Can you work these out from the model? Positions are in its coordinate system, mm. A direction names the side the tool comes from. Coordinates: 2 decimals unless noted, no trailing zeros. Loops run counter-clockwise (first coordinate to the right, second up) from the corner with the lowest first, then second, coordinate; pieces in that order, holes last.
```python
from build123d import *

# Parameters (mm, degrees)
SKETCH1_R                             = 31.75
BOSS_EXTRUDE1_DEPTH                   = 15.24
FILLET1_R                             = 5.08
CUT_EXTRUDE2_DEPTH                    = 74.66
F_1_4_0_26_DIAMETER_HOLE1_D           = 6.604
F_1_4_0_26_DIAMETER_HOLE1_DEPTH       = 25.4
F_1_4_0_26_DIAMETER_HOLE1_CSINK_D     = 12.7
F_1_4_0_26_DIAMETER_HOLE1_CSINK_ANGLE = 100
SKETCH5_R                             = 35.56
CUT_EXTRUDE3_DEPTH                    = 11.43


with BuildPart() as part:
    # Sketch1 → Boss-Extrude1 (new body, symmetric)
    with BuildSketch(Plane.XY):
        with BuildLine():
            Line((-101.6, -54.61), (101.6, -54.61))
            Line((101.6, -54.61), (101.6, -29.21))
            Line((101.6, -29.21), (76.557273058, -29.21))
            ThreePointArc((76.557273058, -29.21), (67.399896086, -26.670434606), (60.858464857, -19.777204386))
            Line((60.858464857, -19.777204386), (39.247020503, 20.868010966))
            ThreePointArc((39.247020503, 20.868010966), (0, 44.45), (-39.247020503, 20.868010966))
            Line((-39.247020503, 20.868010966), (-60.858464857, -19.777204386))
            ThreePointArc((-60.858464857, -19.777204386), (-67.399896086, -26.670434606), (-76.557273058, -29.21))
            Line((-76.557273058, -29.21), (-101.6, -29.21))
            Line((-101.6, -29.21), (-101.6, -54.61))
        make_face()
        Circle(SKETCH1_R, mode=Mode.SUBTRACT)
    extrude(amount=BOSS_EXTRUDE1_DEPTH, both=True)

    # Fillet1
    fillet1_edges = [part.edges().sort_by_distance(p)[0] for p in [
        (101.6, -41.91, 15.24),
        (101.6, -41.91, -15.24),
        (-101.6, -41.91, -15.24),
        (-101.6, -41.91, 15.24),
    ]]
    fillet(fillet1_edges, radius=FILLET1_R)

    # Sketch2 → Cut-Extrude2 (cut, through all)
    with BuildSketch(Plane(origin=(0, -29.21, 0), x_dir=(1, 0, 0), z_dir=(0, 1, 0))):
        with BuildLine():
            Line((-93.98, 11.43), (-60.96, 11.43))
            ThreePointArc((-60.96, 11.43), (-49.53, 0), (-60.96, -11.43))
            Line((-60.96, -11.43), (-93.98, -11.43))
            Line((-93.98, -11.43), (-93.98, 11.43))
        make_face()
        with BuildLine():
            Line((93.98, 11.43), (93.98, -11.43))
            Line((93.98, -11.43), (60.96, -11.43))
            ThreePointArc((60.96, -11.43), (49.53, 0), (60.96, 11.43))
            Line((60.96, 11.43), (93.98, 11.43))
        make_face()
    extrude(amount=CUT_EXTRUDE2_DEPTH, mode=Mode.SUBTRACT)

    # 1/4 (0.26) Diameter Hole1
    with Locations(Plane(origin=(0, -29.21, 0), x_dir=(1, 0, 0), z_dir=(0, 1, 0))):
        with Locations((-69.85, 0), (69.85, 0)):
            CounterSinkHole(F_1_4_0_26_DIAMETER_HOLE1_D / 2, F_1_4_0_26_DIAMETER_HOLE1_CSINK_D / 2, depth=F_1_4_0_26_DIAMETER_HOLE1_DEPTH, counter_sink_angle=F_1_4_0_26_DIAMETER_HOLE1_CSINK_ANGLE)

    # Sketch5 → Cut-Extrude3 (cut, symmetric)
    with BuildSketch(Plane.XY):
        Circle(SKETCH5_R)
    extrude(amount=CUT_EXTRUDE3_DEPTH, both=True, mode=Mode.SUBTRACT)


solid = part.part
```
Item 1: Suppose I cut it at A-A, the plane z = 0. Please give me the cut outline in (x, y), plus the area to 3 significant figures.
Results are:
outline: (-101.6, -54.61) - (-73.15, -54.61) - (-73.15, -31.77) - (-76.2, -29.21) - (-101.6, -29.21) - close; (-66.55, -54.61) - (66.55, -54.61) - (66.55, -31.77) - (63.5, -29.21) - (49.53, -29.21) - (49.53, 1.53) - (39.25, 20.87) arc R44.45 ccw to (-39.25, 20.87) - (-49.53, 1.53) - (-49.53, -29.21) - (-63.5, -29.21) - (-66.55, -31.77) - close; (73.15, -54.61) - (101.6, -54.61) - (101.6, -29.21) - (76.2, -29.21) - (73.15, -31.77) - close; hole circle Ø71.12 at (0, 0)
area: 6,920 mm2
Item 2: Suppose I cut it at B-B, the plane y = 11.5. Please give me the cut outline in (x, z), plus the area to 3 significant figures.
Results are:
outline: (-44.23, -15.24) - (-29.59, -15.24) - (-29.59, -11.43) - (-33.65, -11.43) - (-33.65, 11.43) - (-29.59, 11.43) - (-29.59, 15.24) - (-44.23, 15.24) - close; (29.59, -15.24) - (44.23, -15.24) - (44.23, 15.24) - (29.59, 15.24) - (29.59, 11.43) - (33.65, 11.43) - (33.65, -11.43) - (29.59, -11.43) - close
area: 707 mm2
Item 3: We'd pull the mould along X, two halves only. Please class faces 6 (the face through (-73, -43.35, -0.99)), 7 (the face through (-47.5, 5.35, 0.21)), 8 (the face through (65, -27, -11.43)): +X half, -X half, draft (parallel to the pull), parting line (faces both ways), or undercut.
Results are:
face 6: undercut
face 7: -X half
face 8: draft
Item 4: I need wall thicknesses on line 1 along Y through (x, z) = (0, 13.35); line 2 along Y through (x, z) = (0, 0); line 3 along Y through (x, z) = (-60, -9.5). Which ranges of each line are inside material? Lowest first, please.
Results are:
line 1: y = -54.61 to -31.75, 31.75 to 44.45
line 2: y = -54.61 to -35.56, 35.56 to 44.45
line 3: y = -54.61 to -29.21
Item 5: I'm going to push flat-ended pins straight in: P1, Ø4.5, axis at x = 71.5, y = -25.5, coming from the +Z side; P2, Ø3, axis at x = 69, y = -26.5, coming from the -Z side; P3, Ø1, axis at y = -13.5, z = -10, coming from the -X side; P4, Ø1.5, axis at x = -26.5, z = 4.5, coming from the +Y side. Where does each tip first touch, or does it pass through?
Results are:
P1: passes through
P2: stops at z = -15.24
P3: stops at x = -56.44
P4: stops at y = 36.23
Item 6: Suppose I cut it at D-D, the plane x = -83.5. Please give me the cut outline in (y, z), plus the area to 3 significant figures.
Results are:
outline: (-54.61, -15.24) - (-29.21, -15.24) - (-29.21, 15.24) - (-54.61, 15.24) - close
area: 774 mm2
Item 7: On a 3-axis mill with a long thin cutter (end or side, diameter ignored), from which of +Z, -Z, +X, -X, +Y, -Y can I reach the whole of each face in a straight line? I mean faces 1 (the face through (-13.3, 29.1, 11.43)), 2 (the face through (100.072, -41.732, 13.791)), 3 (the face through (0.673, 44.445, 0.213)), 4 (the face through (65, -27, 11.43)), 5 (the face through (-65, -27, -11.43)). Say none if no direction works.
Results are:
face 1: none
face 2: +Z, +X, +Y, -Y
face 3: +Z, -Z, +Y
face 4: +X, +Y
face 5: -X, +Y
Item 8: Suppose I cut it at C-C, the plane x = 19.5. Please give me the cut outline in (y, z), plus the area to 3 significant figures.
Results are:
outline: (-54.61, -15.24) - (-25.06, -15.24) - (-25.06, -11.43) - (-29.74, -11.43) - (-29.74, 11.43) - (-25.06, 11.43) - (-25.06, 15.24) - (-54.61, 15.24) - close; (25.06, -15.24) - (39.94, -15.24) - (39.94, 15.24) - (25.06, 15.24) - (25.06, 11.43) - (29.74, 11.43) - (29.74, -11.43) - (25.06, -11.43) - close
area: 1,140 mm2
